from build123d import *

# Parameters (mm, degrees)
SKETCH2_W           = 24
SKETCH2_H           = 10
BOSS_EXTRUDE1_DEPTH = 4
SKETCH3_R           = 1.75
CUT_EXTRUDE1_DEPTH  = 5
FILLET1_R           = 1
CUT_EXTRUDE2_DEPTH  = 30


with BuildPart() as part:
    # Sketch2 → Boss-Extrude1 (new body)
    with BuildSketch(Plane.XY):
        with Locations((6.957345972, -1)):
            Rectangle(SKETCH2_W, SKETCH2_H)
    extrude(amount=BOSS_EXTRUDE1_DEPTH)

    # Sketch3 → Cut-Extrude1 (cut)
    with BuildSketch(Plane.XY.offset(4)):
        with Locations((6.957345972, -1)):
            Circle(SKETCH3_R)
    extrude(amount=-CUT_EXTRUDE1_DEPTH, mode=Mode.SUBTRACT)

    # Fillet1
    fillet1_edges = [part.edges().sort_by_distance(p)[0] for p in [
        (6.957345972, 4, 0),
        (6.957345972, -6, 0),
    ]]
    fillet(fillet1_edges, radius=FILLET1_R)

    # Sketch4 → Cut-Extrude2 (cut)
    with BuildSketch(Plane.ZY.offset(5.042654028)):
        with BuildLine():
            ThreePointArc((4, -3.9), (5.025304833, -3.475304833), (5.45, -2.45))
            ThreePointArc((5.45, -2.45), (5.025304832, -1.424695167), (3.999999998, -1))
            Line((4, -1), (4, -3.9))
        make_face()
        with BuildLine():
            Line((4, -3.9), (4, -1))
            ThreePointArc((3.999999998, -1), (2.55, -2.450000001), (4, -3.9))
        make_face()
        with BuildLine():
            ThreePointArc((4, 1.9), (2.55, 0.450000001), (3.999999998, -1))
            Line((4, -1), (4, 1.9))
        make_face()
        with BuildLine():
            Line((4, 1.9), (4, -1))
            ThreePointArc((3.999999998, -1), (5.025304832, -0.575304833), (5.45, 0.45))
            ThreePointArc((5.45, 0.45), (5.025304833, 1.475304833), (4, 1.9))
        make_face()
    extrude(amount=-CUT_EXTRUDE2_DEPTH, mode=Mode.SUBTRACT)


solid = part.part
Geometry check sheet. Reference: the model listing, model coordinates, mm. Give positions to 0.01 mm unless a question says otherwise; leave off trailing zeros. Loops run counter-clockwise (first coordinate to the right, second up) from the corner with the lowest first, then second, coordinate; pieces in that order, holes last. Notation, with made-up numbers: M 54,-16 L 87,-16 A34 ccw 87,14 Z; hole C 18.5,3 d8. An arc over 180 degrees is marked long. Answer as a JSON object with one key per item and string values. Group by question number.
Item 1: Mould release check, pull along Y, two halves, no side actions. Record for faces 1 (the cylindrical face through (5.21, -0.92, 1.58)), 2 (the flat face through (7, -6, 2)), 3 (the cylindrical face through (6.79, 0.98, 2.65)), 4 (the flat face through (7, 1, 0)): pulls with the +Y half, pulls with the -Y half, needs draft (parallel to the pull), parting line crosses it, or undercut.
Item 2: Sectioned sample at D-D on z = 2.3. Record the boundary of the cut face in (x, y), plus the area to 3 significant figures.
Item 3: Sectioned sample at A-A on y = 0.45. Record the boundary of the cut face in (x, z), plus the area to 3 significant figures.
Item 4: Material ranges on L1, parallel to X at y = -1, z = 2.2; L2, parallel to Y at x = -0.25, z = 2.7; L3, parallel to Z at x = 16.5, y = 0.5, recorded low to high.
Item 5: Sectioned sample at C-C on x = 10. Record the boundary of the cut face in (y, z), plus the area to 3 significant figures.
Item 6: Gauge pin test, flat end, axial feed: pin 1 (3 mm diameter, centred on x = 6.96, y = -1, fed in from +Z). Record the tip position at first contact, or that the pin passes through.
Item 7: Sectioned sample at B-B on z = 3.5. Record the boundary of the cut face in (x, y), plus the area to 3 significant figures.
Findings below:
{
 "1": {"face 1": "undercut", "face 2": "pulls with the -Y half", "face 3": "undercut", "face 4": "needs draft"},
 "2": {"outline": "M -5.04,-6 L 18.96,-6 L 18.96,4 L -5.04,4 Z; hole C 6.96,-1 d3.5", "area": "230 mm2"},
 "3": {"outline": "M -5.04,0 L 5.98,0 L 5.98,2.55 L -5.04,2.55 Z; M 7.94,0 L 18.96,0 L 18.96,2.55 L 7.94,2.55 Z", "area": "56.2 mm2"},
 "4": {"L1": "-5.04 to 5.21, 8.71 to 18.96", "L2": "-6 to -3.09, -1.81 to -0.19, 1.09 to 4", "L3": "0 to 2.55"},
 "5": {"outline": "M -6,1 A1 ccw -5,0 L 3,0 A1 ccw 4,1 L 4,4 L 1.9,4 A1.45 cw -1,4 A1.45 cw -3.9,4 L -6,4 Z", "area": "33.0 mm2"},
 "6": {"pin 1": "through"},
 "7": {"outline": "M -5.04,-6 L 18.96,-6 L 18.96,-3.81 L -5.04,-3.81 Z; M -5.04,-1.09 L 5.21,-1.09 A1.75 cw 5.21,-0.91 L -5.04,-0.91 Z; M -5.04,1.81 L 18.96,1.81 L 18.96,4 L -5.04,4 Z; M 8.71,-1.09 L 18.96,-1.09 L 18.96,-0.91 L 8.71,-0.91 A1.75 cw Z", "area": "109 mm2"}
}
